from build123d import *

# Parameters (mm, degrees)
SKETCH1_W             = 60
SKETCH1_H             = 110
BOSS_EXTRUDE1_DEPTH   = 3
FILLET2_R             = 10
M3_CLEARANCE_HOLE1_D  = 3.4
DELETEFACE1_OUTLINE_R = 1.7
DELETEFACE1_DEPTH     = 3
SKETCH6_W             = 5
SKETCH6_H             = 1.8
CUT_EXTRUDE3_DEPTH    = 63.721607122


# Read off the part's stored shape, not the designer's step: DeleteFace1
with BuildPart() as part:
    # Sketch1 → Boss-Extrude1 (new body)
    with BuildSketch(Plane(origin=(0, 0, 0), x_dir=(1, 0, 0), z_dir=(0, 1, 0))):
        Rectangle(SKETCH1_W, SKETCH1_H)
    extrude(amount=BOSS_EXTRUDE1_DEPTH)

    # Fillet2
    fillet2_edges = [part.edges().sort_by_distance(p)[0] for p in [
        (30, 1.5, 55),
        (-30, 1.5, 55),
        (-30, 1.5, -55),
        (30, 1.5, -55),
    ]]
    fillet(fillet2_edges, radius=FILLET2_R)

    # M3 Clearance Hole1 (through all)
    with Locations(Plane(origin=(0, 3, 0), x_dir=(1, 0, 0), z_dir=(0, 1, 0))):
        with Locations((0, 0), (25, 45.5), (-25, -45.5), (-25, 45.5), (25, -45.5)):
            Hole(M3_CLEARANCE_HOLE1_D / 2)

    # DeleteFace1 outline → DeleteFace1 (add)
    with BuildSketch(Plane(origin=(0, 0, 0), x_dir=(1, 0, 0), z_dir=(0, 1, 0))):
        Circle(DELETEFACE1_OUTLINE_R)
    extrude(amount=DELETEFACE1_DEPTH)

    # Sketch6 → Cut-Extrude3 (cut, through all)
    with BuildSketch(Plane(origin=(0, 3, 0), x_dir=(1, 0, 0), z_dir=(0, 1, 0))):
        with Locations((-4.25, 2.6)):
            Rectangle(SKETCH6_W, SKETCH6_H)
        with Locations((4.25, 2.6)):
            Rectangle(SKETCH6_W, SKETCH6_H)
        with Locations((4.25, 8.6)):
            Rectangle(SKETCH6_W, SKETCH6_H)
        with Locations((-4.25, 8.6)):
            Rectangle(SKETCH6_W, SKETCH6_H)
        with Locations((-4.25, 42.1)):
            Rectangle(SKETCH6_W, SKETCH6_H)
        with Locations((-4.25, 48.1)):
            Rectangle(SKETCH6_W, SKETCH6_H)
        with Locations((4.25, 48.1)):
            Rectangle(SKETCH6_W, SKETCH6_H)
        with Locations((4.25, 42.1)):
            Rectangle(SKETCH6_W, SKETCH6_H)
    extrude(amount=-CUT_EXTRUDE3_DEPTH, mode=Mode.SUBTRACT)


solid = part.part
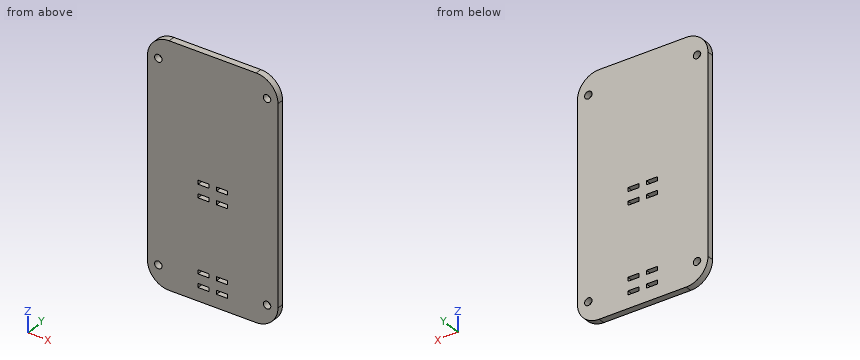
Here's how the part is built. I have some questions about the finished solid (model axes, mm). Coordinates: 2 decimals unless noted, no trailing zeros. Loops run counter-clockwise (first coordinate to the right, second up) from the corner with the lowest first, then second, coordinate; pieces in that order, holes last. Notation, with made-up numbers: (-12, 65) -> (14, 65) arc R31 cw to (14, 104) -> close; hole circle Ø7 at (23.25, 71). An arc over 180 degrees is marked (long way). Use one line per item in the form item = value. Start each with the question number.
(1) If we section it at A-A (x = 24.5): Please give me the cut outline in (y, z), then the cut area to 3 significant figures.
(2) Please list where these lines run through material, in increasing order: line 1 along X through (y, z) = (1.1, 45.5); line 2 along Z through (x, y) = (5, 1.05); line 3 along X through (y, z) = (2.6, -42).
(3) If we section it at B-B (y = 1.8): Give the number of separate pieces and of enclosed holes in the cut face, then the cut area to 3 significant figures.
(4) Will this pin go through, and if not, where does the flat tip stop? pin 1 (0.9 mm diameter, centred on y = 1.5, z = -47.5, fed in from -X).
(5) If we section it at C-C (x = -25): Please give me the cut outline in (y, z).
Verdict:
q1.outline = (0, -53.93) -> (3, -53.93) -> (3, -47.12) -> (0, -47.12) -> close; (0, -43.88) -> (3, -43.88) -> (3, 43.88) -> (0, 43.88) -> close; (0, 47.12) -> (3, 47.12) -> (3, 53.93) -> (0, 53.93) -> close
q1.area = 304 mm²
q2.line_1 = -29.99 to -26.7, -23.3 to 23.3, 26.7 to 29.99
q2.line_2 = -55 to -49, -47.2 to -43, -41.2 to -9.5, -7.7 to -3.5, -1.7 to 55
q2.line_3 = -30 to -6.75, -1.75 to 1.75, 6.75 to 30
q3.separate_pieces = 1
q3.enclosed_holes = 12
q3.area = 6,410 mm²
q4.pin_1 = -29.79
q5.outline = (0, -53.66) -> (3, -53.66) -> (3, -47.2) -> (0, -47.2) -> close; (0, -43.8) -> (3, -43.8) -> (3, 43.8) -> (0, 43.8) -> close; (0, 47.2) -> (3, 47.2) -> (3, 53.66) -> (0, 53.66) -> close
